Autodesk Inventor part; units mm, degrees
ref_plane "YZ Plane" through (0, 0, 0) normal (1, 0, 0) x (0, 1, 0)
ref_plane "XZ Plane" through (0, 0, 0) normal (0, 1, 0) x (-1, 0, 0)
ref_plane "XY Plane" through (0, 0, 0) normal (0, 0, 1) x (1, 0, 0)
sketch "Sketch1" plane through (0, 0, 0) normal (0, 0, 1) x (1, 0, 0)
  line L0 (0, 0) -> (164.5, 0)
  line L1 (164.5, 0) -> (164.5, 9)
  line L2 (164.5, 9) -> (0, 9)
  line L3 (0, 9) -> (0, 0)
  circle A0 centre (57, 4) radius 1.6
  circle A1 centre (99, 4) radius 1.6
  circle A2 centre (159.5, 4) radius 1.6
  circle A3 centre (147, 4) radius 1.6
  circle A4 centre (15, 4) radius 1.6
  circle A5 centre (5, 4) radius 1.6
  dimension "d1" = 9
  dimension "d2" = 90
  dimension "d4" = 3.2
  dimension "d6" = 3.2
  dimension "d7" = 3.2
  dimension "d8" = 42
  dimension "d9" = 60.5
  dimension "d26" = 3.2
  dimension "d27" = 48
  dimension "d28" = 3.2
  dimension "d29" = 42
  dimension "d32" = 15
  dimension "d33" = 5
  dimension "d61" = 3.2
  dimension "d62" = 10
  dimension "d63" = 12.5
  dimension "d108" = 4
  dimension "d109" = 4
  dimension "d110" = 4
  dimension "d111" = 4
  dimension "d112" = 4
  dimension "d113" = 4
ref_plane "Work Plane2" through (0, 0, 0) normal (0, -1, 0) x (1, 0, 0)
sketch "Sketch2" plane through (0, 0, 0) normal (0, -1, 0) x (1, 0, 0)
  circle A0 centre (52, 8) radius 1.6
  circle A1 centre (125, 8) radius 1.6
  circle A2 centre (88.5, 8) radius 1.6
  point P0 (0, 0)
  point P1 (52, 0)
  dimension "d13" = 3.2
  dimension "d15" = 3.2
  dimension "d17" = 3.2
  dimension "d18" = 36.5
  dimension "d64" = 52
  dimension "d65" = 36.5
  dimension "d114" = 8
  dimension "d115" = 73
ref_plane "Work Plane1" through (0, 0, 11) normal (0, 0, 1) x (1, 0, 0)
extrude "klocek" add sketch "Sketch1" along normal blind 11
ref_plane "Work Plane3" through (0, 0, 0) normal (0, -1, 0) x (1, 0, 0)
extrude "prowadzenie osi" cut sketch "Sketch2" against normal up to next
ref_plane "Work Plane4" through (0, 0, 0) normal (0, -1, 0) x (1, 0, 0)
sketch "Sketch7" plane through (0, 0, 0) normal (0, -1, 0) x (1, 0, 0)
  line L0 (0, 11) -> (0, 0)
  line L1 (0, 11) -> (164.5, 11)
  line L2 (0, 11) -> (40, 11)
  line L3 (40, 11) -> (0, 0)
  point P0 (0, -1.8333)
  dimension "d86" = 11
  dimension "d87" = 40
sketch "Sketch8" plane through (0, 0, 0) normal (0, -1, 0) x (1, 0, 0)
  line L0 (164.5, 0) -> (164.5, 11)
  line L1 (164.5, 11) -> (164.5, 3)
  line L2 (164.5, 11) -> (0, 11)
  line L3 (164.5, 11) -> (134.5, 11)
  line L4 (134.5, 11) -> (164.5, 3)
  point P0 (0, 0)
  point P1 (40.8333, 11)
  dimension "d80" = 8
  dimension "d81" = 30
extrude "przedni skos" cut sketch "Sketch7" against normal up to next
extrude "tylni skos" cut sketch "Sketch8" against normal up to next
ref_plane "Work Plane7" through (0, 0, 11) normal (0, 0, 1) x (1, 0, 0)
sketch "Sketch5" plane through (0, 0, 11) normal (0, 0, 1) x (1, 0, 0)
  circle A0 centre (99, 4) radius 1.6
  line L0 (95.5936, 4) -> (97.2968, 6.95)
  line L1 (97.2968, 6.95) -> (100.7032, 6.95)
  line L2 (100.7032, 6.95) -> (102.4064, 4)
  line L3 (102.4064, 4) -> (100.7032, 1.05)
  line L4 (100.7032, 1.05) -> (97.2968, 1.05)
  line L5 (97.2968, 1.05) -> (95.5936, 4)
  circle A1 centre (57, 4) radius 1.6
  line L6 (60.4064, 4) -> (58.7032, 1.05)
  line L7 (58.7032, 1.05) -> (55.2968, 1.05)
  line L8 (55.2968, 1.05) -> (53.5936, 4)
  line L9 (53.5936, 4) -> (55.2968, 6.95)
  line L10 (55.2968, 6.95) -> (58.7032, 6.95)
  line L11 (58.7032, 6.95) -> (60.4064, 4)
  point P0 (119.5, 5)
  dimension "d98" = 5.9
  dimension "d100" = 5.9
extrude "hex insert middle" cut sketch "Sketch5" against normal blind 3
ref_plane "Work Plane6" through (0, 0, 11) normal (0, 0, 1) x (1, 0, 0)
sketch "Sketch9" plane through (0, 0, 11) normal (0, 0, 1) x (1, 0, 0)
  circle A0 centre (147, 4) radius 1.6
  line L0 (150.4064, 4) -> (148.7032, 1.05)
  line L1 (148.7032, 1.05) -> (145.2968, 1.05)
  line L2 (145.2968, 1.05) -> (143.5936, 4)
  line L3 (143.5936, 4) -> (145.2968, 6.95)
  line L4 (145.2968, 6.95) -> (148.7032, 6.95)
  line L5 (148.7032, 6.95) -> (150.4064, 4)
  point P0 (0, 0)
  point P1 (153, 5)
  dimension "d99" = 5.9
extrude "hex insert rear 1" cut sketch "Sketch9" against normal blind 6.5
ref_plane "Work Plane5" through (0, 0, 11) normal (0, 0, 1) x (1, 0, 0)
sketch "Sketch10" plane through (0, 0, 11) normal (0, 0, 1) x (1, 0, 0)
  circle A0 centre (159.5, 4) radius 1.6
  line L0 (162.9064, 4) -> (161.2032, 1.05)
  line L1 (161.2032, 1.05) -> (157.7968, 1.05)
  line L2 (157.7968, 1.05) -> (156.0936, 4)
  line L3 (156.0936, 4) -> (157.7968, 6.95)
  line L4 (157.7968, 6.95) -> (161.2032, 6.95)
  line L5 (161.2032, 6.95) -> (162.9064, 4)
  point P0 (0, 0)
  dimension "d101" = 5.9
extrude "hex insert rear 2" cut sketch "Sketch10" against normal blind 8.5
sketch "Sketch13" plane through (0, 0, 11) normal (0, 0, 1) x (1, 0, 0)
  line L0 (197.4, 0) -> (-32.9, 0)
  line L1 (7.95, 2.2968) -> (5, 0.5936)
  line L2 (5, 0.5936) -> (2.05, 2.2968)
  line L3 (2.05, 2.2968) -> (2.05, 5.7032)
  line L4 (2.05, 5.7032) -> (5, 7.4064)
  line L5 (5, 7.4064) -> (7.95, 5.7032)
  line L6 (7.95, 5.7032) -> (7.95, 2.2968)
  point P0 (0, 0)
  point P1 (5, 4)
  point P2 (5, 4)
  dimension "d117" = 5.9
extrude "hex insert front 1" cut sketch "Sketch13" against normal through all
sketch "Sketch16" plane through (0, 0, 11) normal (0, 0, 1) x (1, 0, 0)
  circle A0 centre (15, 4) radius 1.6
  line L0 (18.4064, 4) -> (16.7032, 1.05)
  line L1 (16.7032, 1.05) -> (13.2968, 1.05)
  line L2 (13.2968, 1.05) -> (11.5936, 4)
  line L3 (11.5936, 4) -> (13.2968, 6.95)
  line L4 (13.2968, 6.95) -> (16.7032, 6.95)
  line L5 (16.7032, 6.95) -> (18.4064, 4)
  point P0 (0, 0)
  dimension "d93" = 5.9
extrude "hex insert front 2" cut sketch "Sketch16" against normal blind 9
sketch "Sketch17" plane through (0, 0, 0) normal (0, 0, -1) x (-1, 0, 0)
  line L0 (0, 9) -> (0, 0)
  line L1 (0, 0) -> (-5, 0)
  line L2 (-5, 0) -> (-5, 10.0042)
  line L3 (-5, 10.0042) -> (0, 10.0042)
  line L4 (0, 10.0042) -> (0, 0)
  point P0 (-5, 7.4064)
extrude "Extrusion20" cut sketch "Sketch17" against normal up to next
sketch "Sketch18" plane through (40, 0, 11) normal (0, -1, 0) x (1, 0, 0)
  line L0 (9.5, 0) -> (9.5, -2)
  line L1 (9.5, -2) -> (-7.5, -2)
  line L2 (-7.5, -2) -> (-7.5, 0)
  line L3 (-7.5, 0) -> (9.5, 0)
  line L4 (94.5, 0) -> (0, 0)
  circle A0 centre (12, -3) radius 1.6
  line L5 (-35, -11) -> (124.5, -11)
  point P0 (-40, -11)
  dimension "d102" = 2
  dimension "d103" = 17
  dimension "d104" = 2.5
extrude "Extrusion21" cut sketch "Sketch18" against normal blind 7.3 contours L0 L1 L2 L3
properties part number "wheel_support_v3_narrow_with_line_sensor_all_holes"
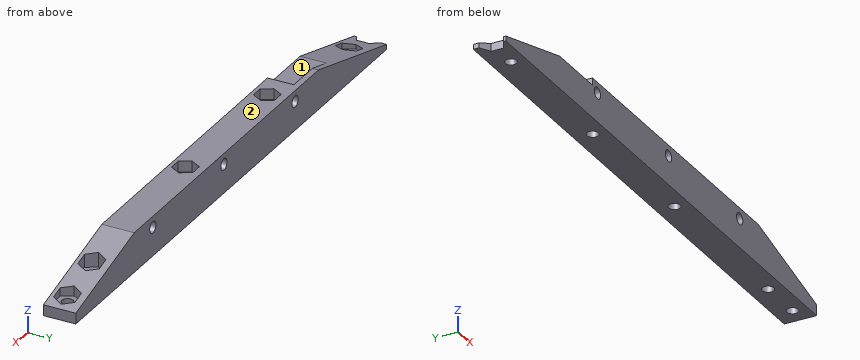
Read the model definition and answer for the solid it produces. Units are mm, in the model's axes. Face numbers are marked on the shaded views. A direction names the side the tool comes from. Give positions to 0.01 mm unless a question says otherwise; leave off trailing zeros. Loops run counter-clockwise (first coordinate to the right, second up) from the corner with the lowest first, then second, coordinate; pieces in that order, holes last.
Item 1: The part is cut by section B-B (x = 147). Write down the section's boundary in (y, z), and give its area (3 significant figures).
Item 2: Find the intervals of material crossed by line 1 along Y through (x, z) = (15, 0.55); line 2 along Z through (x, y) = (88.5, 3.25); line 3 along Z through (x, y) = (45, 4.5), in increasing order.
Item 3: Each of these flat-tipped pins is pushed along its axis until it touches: pin 1 Ø4 at (x, y) = (28.5, 5) entering from +Z; pin 2 Ø3 at (x, y) = (56.5, 5) entering from +Z; pin 3 Ø3.5 at (x, y) = (39, 3) entering from +Z. Where does it stop, or does it pass through?
Item 4: For the marked faces 1 and 2, determine the directions among +Z, -Z, +X, -X, +Y, -Y from which every point of the face is accessible in a straight line to the end or side of a thin tool.
Item 5: The part is cut by section C-C (x = 30.5). Write down the section's boundary in (y, z).
Item 6: The part is cut by section A-A (x = 88.5). Write down the section's boundary in (y, z), and give its area (3 significant figures).
Taken from the geometry:
1. outline: (0, 0) - (2.4, 0) - (2.4, 4.5) - (1.05, 4.5) - (1.05, 7.67) - (0, 7.67) - close; (5.6, 0) - (9, 0) - (9, 7.67) - (6.95, 7.67) - (6.95, 4.5) - (5.6, 4.5) - close
1. area: 35.9 mm2
2. line 1: y = 0 to 2.4, 5.6 to 9
2. line 2: z = 0 to 6.4, 9.6 to 11
2. line 3: z = 0 to 9
3. pin 1: stops at z = 8.39
3. pin 2: stops at z = 8
3. pin 3: stops at z = 9
4. face 1: +Z, -X, -Y
4. face 2: +Z, +X, -X, +Y, -Y
5. outline: (0, 0) - (9, 0) - (9, 8.39) - (0, 8.39) - close
6. outline: (0, 0) - (9, 0) - (9, 6.4) - (0, 6.4) - close; (0, 9.6) - (9, 9.6) - (9, 11) - (0, 11) - close
6. area: 70.2 mm2
